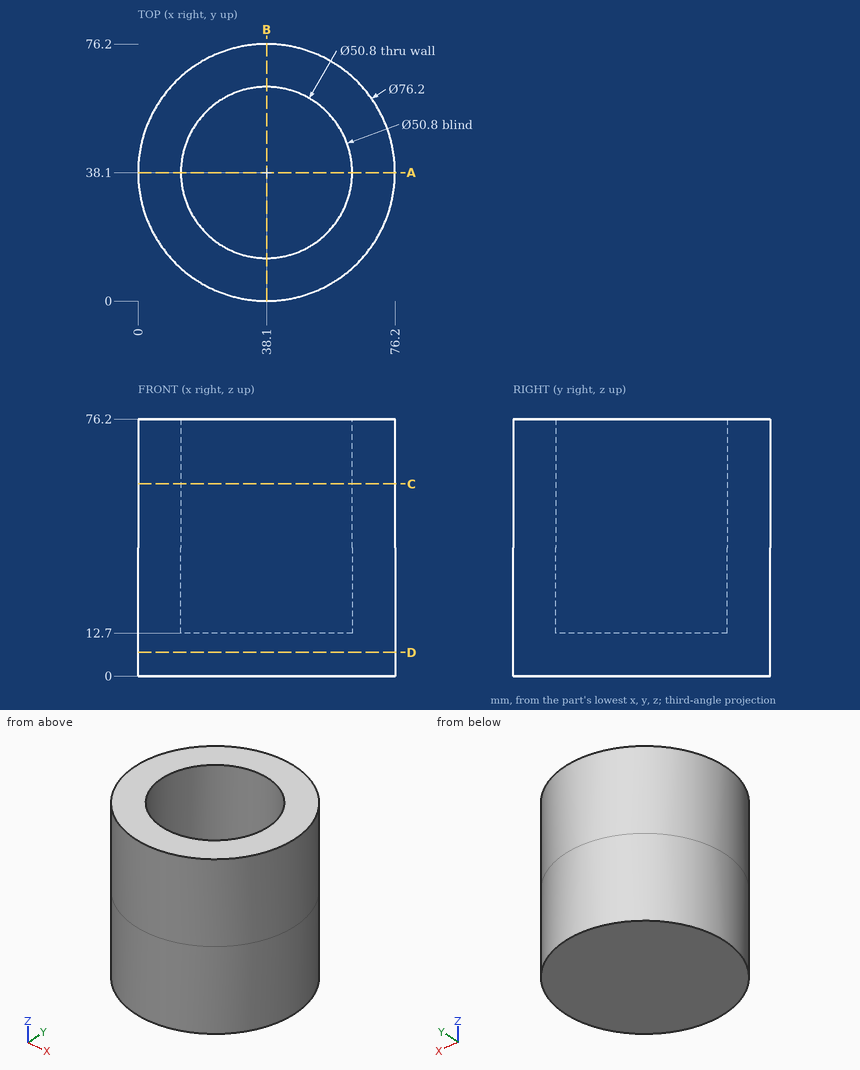
Input: dimensioned drawing with shaded views. Units: mm. Origin: part minimum x, y, z. Give positions to 0.01 mm unless a question says otherwise; leave off trailing zeros. Write each loop counter-clockwise with the first axis right and the second up, starting at its lowest first coordinate (ties: lowest second). Pieces come first, ordered by that corner, then holes.
1. Section query C-C, the plane z = 57. Return loops of the section in (x, y).
2. Section query A-A, the plane y = 38.1. Return loops of the section in (x, z).
3. Pin query (flat end, axial travel): P1, Ø5, axis at x = 32.5, y = 53.5, coming from the -Z side; P2, Ø3, axis at x = 41, y = 43, coming from the +Z side; P3, Ø10, axis at y = 44, z = 53, coming from the -X side; P4, Ø10, axis at y = 61, z = 55.5, coming from the -X side. Return the tip coordinate at first contact, or that it passes through.
4. Line query: probe 1 along Y at (x, z) = (38, 60); probe 2 along Z at (x, y) = (29, 20); probe 3 along Y at (x, z) = (32, 26). Output: solid intervals per line, ascending.
5. Section query D-D, the plane z = 7. Return loops of the section in (x, y), then the cut area to 3 significant figures.
Computed:
1. outline: circle Ø76.2 at (38.1, 38.1); hole circle Ø50.8 at (38.1, 38.1)
2. outline: (0, 0) - (76.2, 0) - (76.2, 76.2) - (63.5, 76.2) - (63.5, 12.7) - (12.7, 12.7) - (12.7, 76.2) - (0, 76.2) - close
3. P1: stops at z = 0
3. P2: stops at z = 12.7
3. P3: stops at x = 0.01
3. P4: stops at x = 4.47
4. probe 1: y = 0 to 12.7, 63.5 to 76.2
4. probe 2: z = 0 to 12.7
4. probe 3: y = 0.49 to 13.44, 62.76 to 75.71
5. outline: circle Ø76.2 at (38.1, 38.1)
5. area: 4,560 mm2
